```python
from build123d import *

# Parameters (mm, degrees)
SKETCH_1_W           = 36
SKETCH_1_H           = 10
EXTRUDE_1_DEPTH      = 70
EXTRUDE_2_DEPTH      = 5
EXTRUDE_2_DEPTH_BACK = 5


with BuildPart() as part:
    # 草图1 → 凸台-拉伸1 (new body)
    with BuildSketch(Plane(origin=(0, 0, 1023.154259328), x_dir=(-1, 0, 0), z_dir=(0, 0, -1))):
        with Locations((86.606649797, -103.783530386)):
            Rectangle(SKETCH_1_W, SKETCH_1_H)
    extrude(amount=EXTRUDE_1_DEPTH)

    # 草图3 → 凸台-拉伸2 (add, two sides: drawn at the far end of the back side and taken through both)
    with BuildSketch(Plane.ZY.offset(86.606649797).offset(-EXTRUDE_2_DEPTH_BACK)):
        Polygon((953.154259328, -98.783530386), (953.154259328, -78.783530386), (973.154259328, -98.783530386), align=None)
    extrude(amount=EXTRUDE_2_DEPTH + EXTRUDE_2_DEPTH_BACK)


solid = part.part
```
For this review, take the finished solid that the model builds, in its own axes (mm). A direction names the side the tool comes from. Give positions to 0.01 mm unless a question says otherwise; leave off trailing zeros. Write each loop counter-clockwise with the first axis right and the second up, starting at its lowest first coordinate (ties: lowest second). Pieces come first, ordered by that corner, then holes. Notation, with made-up numbers: M 16,-34 L 39,-34 A28 cw 39,-2 Z; hole C -28,5.5 d6. An arc over 180 degrees is marked long. One line per item, written item: value.
1) For P1, Ø8, axis at x = -76, y = -88.5, coming from the -Z side; P2, Ø16, axis at y = -88, z = 963.5, coming from the -X side; P3, Ø18, axis at x = -95, z = 999, coming from the +Y side; P4, Ø6, axis at x = -90, y = -86, coming from the +Z side, all flat-tipped, find the tip position at first contact; note any pin that passes through.
Results are:
P1: passes through
P2: stops at x = -91.61
P3: stops at y = -98.78
P4: stops at z = 963.37
2) Take a section at A-A, the plane z = 960. Write out the cut boundary in (x, y).
Results are:
outline: M -104.61,-108.78 L -68.61,-108.78 L -68.61,-98.78 L -81.61,-98.78 L -81.61,-85.63 L -91.61,-85.63 L -91.61,-98.78 L -104.61,-98.78 Z
3) For line 1 (X direction, y = -97.5, z = 958.5); line 2 (Y direction, x = -80, z = 988); line 3 (Z direction, x = -82.5, y = -83.75), list the stretches that pass through material, from the lowest coordinate up. Write a range as from..to.
Results are:
line 1: x = -91.61..-81.61
line 2: y = -108.78..-98.78
line 3: z = 953.15..958.12
4) Take a section at C-C, the plane y = -91. Write out the cut boundary in (x, z), then the cut area to 3 significant figures.
Results are:
outline: M -91.61,953.15 L -81.61,953.15 L -81.61,965.37 L -91.61,965.37 Z
area: 122 mm²
5) For faces 1 (the flat face through (-91.607, -93, 959)), 2 (the flat face through (-68.607, -104, 989)), 3 (the flat face through (-86, -98.784, 989)), 4 (the flat face through (-81.607, -93, 959)), 5 (the flat face through (-104.607, -104, 989)), list the 3-axis set-ups (+Z, -Z, +X, -X, +Y, -Y) from which the entire face can be reached by the end or side of a thin tool; tool diameter is ignored.
Results are:
face 1: +Z, -Z, -X, +Y
face 2: +Z, -Z, +X, +Y, -Y
face 3: +Z, +Y
face 4: +Z, -Z, +X, +Y
face 5: +Z, -Z, -X, +Y, -Y
6) Take a section at D-D, the plane z = 968.5. Write out the cut boundary in (x, y), then the cut area to 3 significant figures.
Results are:
outline: M -104.61,-108.78 L -68.61,-108.78 L -68.61,-98.78 L -81.61,-98.78 L -81.61,-94.13 L -91.61,-94.13 L -91.61,-98.78 L -104.61,-98.78 Z
area: 407 mm²
7) Take a section at B-B, the plane x = -84. Write out the cut boundary in (y, z).
Results are:
outline: M -108.78,953.15 L -78.78,953.15 L -98.78,973.15 L -98.78,1023.15 L -108.78,1023.15 Z
